The drawing under review shows one solid part. Ordinate dimensions are in mm from its lowest x, y, z. Coordinates: 2 decimals unless noted, no trailing zeros. Write each loop counter-clockwise with the first axis right and the second up, starting at its lowest first coordinate (ties: lowest second). Pieces come first, ordered by that corner, then holes.
Q1. Take a section at A-A (z = 3). Give the boundary of the cut face in (x, y), and give its area (3 significant figures).
Q2. For probe 1 along Z at (x, y) = (4, 0.15); probe 2 along Z at (x, y) = (3.75, 0.25); probe 3 along X at (y, z) = (0.1, 13.5), list the stretches that pass through material, from the lowest coordinate up.
Q3. Take a section at D-D (z = 15). Give the boundary of the cut face in (x, y).
Q4. Take a section at C-C (y = 0.15). Give the boundary of the cut face in (x, z).
Q5. Take a section at B-B (x = 2.75). Give the boundary of the cut face in (y, z).
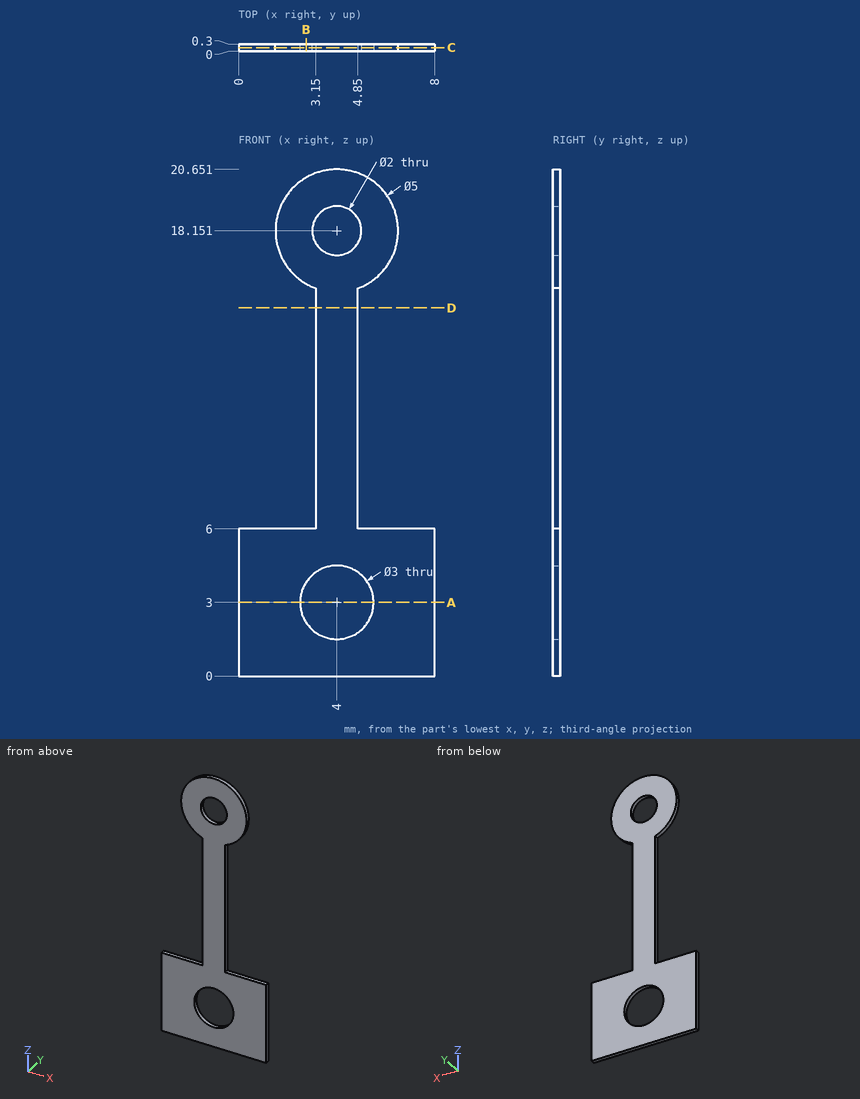
Response:
1. outline: (0, 0) - (2.5, 0) - (2.5, 0.3) - (0, 0.3) - close; (5.5, 0) - (8, 0) - (8, 0.3) - (5.5, 0.3) - close
1. area: 1.50 mm2
2. probe 1: z = 0 to 1.5, 4.5 to 17.15, 19.15 to 20.65
2. probe 2: z = 0 to 1.52, 4.48 to 17.18, 19.12 to 20.64
2. probe 3: x = 3.15 to 4.85
3. outline: (3.15, 0) - (4.85, 0) - (4.85, 0.3) - (3.15, 0.3) - close
4. outline: (0, 0) - (8, 0) - (8, 6) - (4.85, 6) - (4.85, 15.8) arc R2.5 ccw (long way) to (3.15, 15.8) - (3.15, 6) - (0, 6) - close; hole circle Ø3 at (4, 3); hole circle Ø2 at (4, 18.15)
5. outline: (0, 0) - (0.3, 0) - (0.3, 2.17) - (0, 2.17) - close; (0, 3.83) - (0.3, 3.83) - (0.3, 6) - (0, 6) - close; (0, 15.99) - (0.3, 15.99) - (0.3, 20.32) - (0, 20.32) - close
